from build123d import *

# Parameters (mm, degrees)
BOSS_EXTRU_1_DEPTH = 450
ESQUISSE1_3_R      = 7.5
BOSS_EXTRU_2_DEPTH = 350
ESQUISSE1_4_R      = 12.5
ESQUISSE1_4_R_2    = 7.5
BOSS_EXTRU_3_DEPTH = 200


with BuildPart() as part:
    # Esquisse1 → Boss.-Extru.1 (new body)
    with BuildSketch(Plane.XY):
        with BuildLine():
            ThreePointArc((114, 0), (101.5, -12.5), (89, 0))
            ThreePointArc((89, 0), (62.932503523, -62.932503528), (-6e-09, -89))
            ThreePointArc((-6e-09, -89), (8.838834763, -92.661165233), (12.5, -101.5))
            ThreePointArc((12.5, -101.5), (8.838834791, -110.338834739), (7.4e-08, -114))
            ThreePointArc((7.4e-08, -114), (80.610173081, -80.610173029), (114, 0))
        make_face()
    extrude(amount=-BOSS_EXTRU_1_DEPTH)



with BuildPart() as body_2:
    # Esquisse1_3 → Boss.-Extru.2 (new body)
    with BuildSketch(Plane.XY):
        with Locations((101.5, 0)):
            Circle(ESQUISSE1_3_R)
    extrude(amount=-BOSS_EXTRU_2_DEPTH)


with BuildPart() as part_1:
    add(part.part)

    add(body_2.part)  # Boss.-Extru.3 merges body 2
    # Esquisse1_4 → Boss.-Extru.3 (add)
    with BuildSketch(Plane.XY):
        with Locations((101.5, 0)):
            Circle(ESQUISSE1_4_R)
        with Locations((101.5, 0)):
            Circle(ESQUISSE1_4_R_2, mode=Mode.SUBTRACT)
    extrude(amount=-BOSS_EXTRU_3_DEPTH)


solid = part_1.part
Read the model definition and answer for the solid it produces. Units are mm, in the model's axes. A direction names the side the tool comes from. Round coordinates to 2 decimals unless told otherwise and drop trailing zeros. Write each loop counter-clockwise with the first axis right and the second up, starting at its lowest first coordinate (ties: lowest second). Pieces come first, ordered by that corner, then holes.
Q1. Find section D-D on y = -106. Determine the outline of the cut face in (x, z), and give its area (3 significant figures).
Values:
outline: (11.66, -450) - (41.95, -450) - (41.95, 0) - (11.66, 0) - close
area: 13,600 mm2
Q2. The mould has two halves that part along Y. Classify faces 1 (the face through (79.72, -81.49, -221.85)), 2 (the face through (101.775, -12.497, -323.25)), 3 (the face through (74, -55, 0)): released by +Y, released by -Y, zero draft, split by the parting line, or undercut.
Values:
face 1: released by -Y
face 2: undercut
face 3: zero draft
Q3. Find section A-A on z = -89. Determine the outline of the cut face in (x, y), and give its area (3 significant figures).
Values:
outline: (0, -114) arc R114 ccw to (114, 0) arc R12.5 ccw to (89, 0) arc R89 cw to (0, -89) arc R12.5 cw to start
area: 3,990 mm2
Q4. Flat-ended cylindrical pins translate along their axes: P1, Ø12, axis at y = -37, z = -100.5, coming from the -X side; P2, Ø5, axis at y = -43.5, z = -391, coming from the +X side; P3, Ø20, axis at x = 96.5, y = 1.5, coming from the -Z side; P4, Ø3, axis at x = 47.5, z = -92, coming from the +Y side. Find the tip coordinate at first contact, or state that the pin passes through.
Values:
P1: stops at x = 77.92
P2: stops at x = 106.37
P3: stops at z = -450
P4: stops at y = -74.3
Q5. Find section B-B on x = 8.5. Determine the outline of the cut face in (y, z).
Values:
outline: (-113.68, -450) - (-110.67, -450) - (-110.67, 0) - (-113.68, 0) - close; (-92.33, -450) - (-88.59, -450) - (-88.59, 0) - (-92.33, 0) - close
Q6. Straight lines are drawn through the part: line 1 (X direction, y = -3, z = -106.5); line 2 (X direction, y = -18, z = -364.5); line 3 (Y direction, x = 57, z = -42). For each, find the intervals that lie inside material, in ascending order.
Values:
line 1: x = 88.95 to 113.96
line 2: x = 87.16 to 112.57
line 3: y = -98.73 to -68.35
Q7. Find section C-C on x = 101.5. Determine the outline of the cut face in (y, z).
Values:
outline: (-51.9, -450) - (-12.5, -450) - (-12.5, -200) - (-7.5, -200) - (-7.5, -350) - (7.5, -350) - (7.5, -200) - (12.5, -200) - (12.5, 0) - (-51.9, 0) - close
Q8. A tool of negligible diameter and unlimited length cuts with its end or side. For faces 4 (the face through (101, 0, -350)), 5 (the face through (65, -69, -450)), 6 (the face through (94, 0, -274)), from which of +Z, -Z, +X, -X, +Y, -Y can it reach the whole face along a straight path? Write none if from no direction.
Values:
face 4: -Z, +Y
face 5: -Z, +X, -X, +Y, -Y
face 6: -Z
